Build history of the part. All positions in model axes, mm. Face numbers are marked on the shaded views. Give positions to 0.01 mm unless a question says otherwise; leave off trailing zeros. Write each loop counter-clockwise with the first axis right and the second up, starting at its lowest first coordinate (ties: lowest second). Pieces come first, ordered by that corner, then holes. Notation, with made-up numbers: (-12, 84) -> (5, 84) arc R32 ccw to (5, 118) -> close; hole circle Ø2 at (45.25, 55). An arc over 180 degrees is marked (long way). Write item = value, one per line. Start each with the question number.
Q1. Mould opens along X. For the marked faces 1, 2 and 3 say: pulls with the +X half, pulls with the -X half, needs draft (parallel to the pull), parting line crosses it, or undercut.
Q2. Saw through at C-C, the plane y = 4.4. List the corners of the cut face in (x, z).
Q3. Wall check: line 1 (X direction, y = 1.8, z = 0); line 2 (X direction, y = 3.1, z = -1.25); line 3 (Z direction, x = -0.25, y = 4.7). Give the ranges that are in metal, low to high.
Q4. Saw through at D-D, the plane x = -0.75. Give the number of separate pieces and of enclosed holes in the cut face, then the cut area to 3 significant figures.
Q5. Saw through at A-A, the plane y = 3.6. List the corners of the cut face in (x, z), then the cut area to 3 significant figures.
Q6. Saw through at B-B, the plane y = 0.75. List the corners of the cut face in (x, z).
Q7. Drop flat-ended pins along their axis: P1, Ø2.5, axis at x = 0, z = 0, coming from the +Y side (1 decimal); P2, Ø1.5, axis at y = 0.5, z = -2, coming from the -X side. Give the stop position or say it passes through.
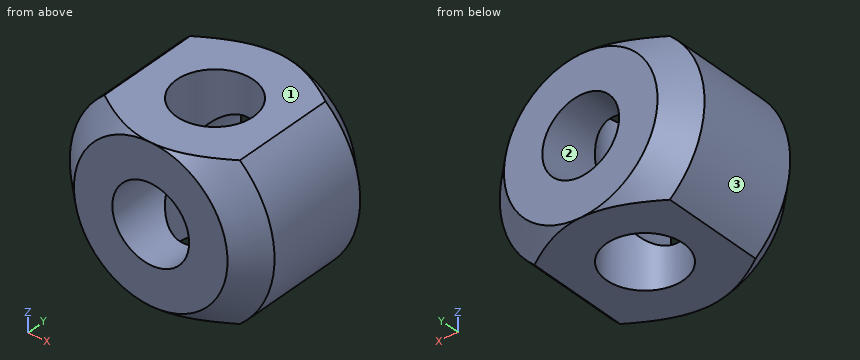
from build123d import *

# Parameters (mm, degrees)
CROQUIS1_R                 = 4
CROQUIS1_R_2               = 1.5
SALIENTE_EXTRUIR3_DEPTH    = 6
CHAFL_N1_SIZE              = 1
CHAFL_N2_SIZE              = 1
CORTAR_EXTRUIR2_DEPTH      = 4
CORTAR_EXTRUIR2_DEPTH_BACK = 4
CROQUIS3_W                 = 2
CROQUIS3_H                 = 6
CROQUIS4_R                 = 1.5
CORTAR_EXTRUIR3_DEPTH      = 6


with BuildPart() as part:
    # Croquis1 → Saliente-Extruir3 (new body)
    with BuildSketch(Plane(origin=(0, 0, 0), x_dir=(1, 0, 0), z_dir=(0, 1, 0))):
        with Locations(Location((0, 0, 0), (0, 0, 270))):
            Circle(CROQUIS1_R)
        with Locations(Location((0, 0, 0), (0, 0, 270))):
            Circle(CROQUIS1_R_2, mode=Mode.SUBTRACT)
    extrude(amount=SALIENTE_EXTRUIR3_DEPTH)

    # Chafl_n1
    chafl_n1_edges = [part.edges().sort_by_distance(p)[0] for p in [
        (0, 6, -4),
    ]]
    chamfer(chafl_n1_edges, length=CHAFL_N1_SIZE)

    # Chafl_n2
    chafl_n2_edges = [part.edges().sort_by_distance(p)[0] for p in [
        (0, 0, -4),
    ]]
    chamfer(chafl_n2_edges, length=CHAFL_N2_SIZE)

    # Croquis3 → Cortar-Extruir2 (cut, two sides: drawn at the far end of the back side and taken through both)
    with BuildSketch(Plane(origin=(0, 0, 0), x_dir=(0, 0, -1), z_dir=(1, 0, 0)).offset(-CORTAR_EXTRUIR2_DEPTH_BACK)):
        with Locations((-4, 3)):
            Rectangle(CROQUIS3_W, CROQUIS3_H)
        with Locations((4, 3)):
            Rectangle(CROQUIS3_W, CROQUIS3_H)
    extrude(amount=CORTAR_EXTRUIR2_DEPTH + CORTAR_EXTRUIR2_DEPTH_BACK, mode=Mode.SUBTRACT)

    # Croquis4 → Cortar-Extruir3 (cut)
    with BuildSketch(Plane.XY.offset(3)):
        with Locations((0, 3)):
            Circle(CROQUIS4_R)
    extrude(amount=-CORTAR_EXTRUIR3_DEPTH, mode=Mode.SUBTRACT)


solid = part.part
Report:
q1.face_1 = needs draft
q1.face_2 = undercut
q1.face_3 = pulls with the -X half
q2.outline = (-2.65, -3) -> (-0.54, -3) -> (-0.54, -1.4) arc R1.5 cw to (-0.54, 1.4) -> (-0.54, 3) -> (-2.65, 3) arc R4 ccw to start; (0.54, -3) -> (2.65, -3) arc R4 ccw to (2.65, 3) -> (0.54, 3) -> (0.54, 1.4) arc R1.5 cw to (0.54, -1.4) -> close
q3.line_1 = -4 to -1.5, 1.5 to 4
q3.line_2 = -3.8 to -1.5, 1.5 to 3.8
q3.line_3 = -3 to -1.48, 1.48 to 3
q4.separate_pieces = 4
q4.enclosed_holes = 0
q4.area = 11.6 mm2
q5.outline = (-2.65, -3) -> (-1.37, -3) -> (-1.37, -0.6) arc R1.5 cw to (-1.37, 0.6) -> (-1.37, 3) -> (-2.65, 3) arc R4 ccw to start; (1.37, -3) -> (2.65, -3) arc R4 ccw to (2.65, 3) -> (1.37, 3) -> (1.37, 0.6) arc R1.5 cw to (1.37, -0.6) -> close
q5.area = 26.3 mm2
q6.outline = (-2.25, -3) -> (2.25, -3) arc R3.75 ccw to (2.25, 3) -> (-2.25, 3) arc R3.75 ccw to start; hole circle Ø3 at (0, 0)
q7.P1 = through
q7.P2 = -3.73
